Autodesk Inventor part; units mm, degrees
ref_plane "YZ Plane" through (0, 0, 0) normal (1, 0, 0) x (0, 1, 0)
ref_plane "XZ Plane" through (0, 0, 0) normal (0, 1, 0) x (-1, 0, 0)
ref_plane "XY Plane" through (0, 0, 0) normal (0, 0, 1) x (1, 0, 0)
sketch "Sketch1" plane through (0, 0, 0) normal (0, 1, 0) x (-1, 0, 0)
  line L0 (13.8415, 5.1768) -> (-89.2585, 5.1768)
  line L1 (-89.2585, 5.1768) -> (-89.2585, -12.8232)
  line L2 (-89.2585, -12.8232) -> (-79.2585, -12.8232)
  line L3 (-79.2585, -12.8232) -> (-79.2585, -4.5732)
  line L4 (-79.2585, -4.5732) -> (-0.8085, -4.5732)
  line L5 (-0.8085, -4.5732) -> (-0.8085, -11.3232)
  line L6 (-0.8085, -11.3232) -> (13.8415, -11.3232)
  line L7 (13.8415, -11.3232) -> (13.8415, 5.1768)
  circle A0 centre (2.4165, -8.8982) radius 1.325
  circle A1 centre (-83.9335, -9.1482) radius 1.325
  line L8 (13.8415, 5.1768) -> (-89.2585, 5.1768)
  line L9 (-89.2585, 5.1768) -> (-89.2585, 6.1768)
  line L10 (-89.2585, 6.1768) -> (13.8415, 6.1768)
  line L11 (13.8415, 6.1768) -> (13.8415, 5.1768)
  point P0 (0, 0)
  dimension "d0" = 2.65
  dimension "d1" = 2.65
  dimension "d2" = 103.1
  dimension "d3" = 14.65
  dimension "d4" = 10
  dimension "d5" = 18
  dimension "d6" = 16.5
  dimension "d7" = 14.075
  dimension "d8" = 11.425
  dimension "d9" = 9.75
  dimension "d10" = 14.325
  dimension "d11" = 5.325
  dimension "d14" = 1
extrude "Extrusion1" add sketch "Sketch1" along normal blind 1
extrude "Extrusion2" add sketch "Sketch1" against normal blind 7.6 contours L0 L9 L10 L11
sketch "Sketch3" plane through (89.2585, 0, 5.1768) normal (0, 0, -1) x (-1, 0, 0)
  line L0 (103.1, -7.6) -> (0, -7.6)
  line L1 (103.1, -7.6) -> (103.1, 1)
  line L2 (0, -7.6) -> (103.1, -7.6)
  line L3 (103.1, -7.6) -> (103.1, -6.6)
  line L4 (103.1, -6.6) -> (0, -6.6)
  line L5 (0, -6.6) -> (0, -7.6)
  point P0 (89.2585, 0)
  dimension "d17" = 1
extrude "Extrusion3" add sketch "Sketch3" along normal blind 19
sketch "Sketch4" plane through (0, 1, 0) normal (0, 1, 0) x (1, 0, 0)
  line L0 (79.2585, 4.5732) -> (0.8085, 4.5732)
  line L1 (18.2585, 4.5732) -> (33.2585, 4.5732)
  line L2 (33.2585, 4.5732) -> (33.2585, 0.3232)
  line L3 (33.2585, 0.3232) -> (18.2585, 0.3232)
  line L4 (18.2585, 0.3232) -> (18.2585, 4.5732)
  line L5 (0.8085, 4.5732) -> (0.8085, 11.3232)
  line L6 (79.2585, 12.8232) -> (79.2585, 4.5732)
  line L7 (-13.8415, -6.1768) -> (89.2585, -6.1768)
  point P0 (0, 0)
  point P1 (33.2585, 4.5732)
  dimension "d21" = 15
  dimension "d26" = 6.5
  dimension "d28" = 46
extrude "Extrusion4" cut sketch "Sketch4" against normal blind 2
properties part number "CO-1-03-jetsonMount"
Part model, mm, in its own coordinate system. A direction names the side the tool comes from. Round coordinates to 2 decimals unless told otherwise and drop trailing zeros. Loops run counter-clockwise (first coordinate to the right, second up) from the corner with the lowest first, then second, coordinate; pieces in that order, holes last. Notation, with made-up numbers: (-3.75, 47) - (5.25, 47) arc R26 cw to (5.25, 83) - close; hole circle Ø1 at (88.5, 19). An arc over 180 degrees is marked (long way). Answer as a JSON object with one key per item and string values.
Item 1: Pull direction Y, two halves, no side cores. Call faces 1 (the face through (38, 0, 0)), 2 (the face through (37, -6.6, -4)), 3 (the face through (38, 1, 1)), 4 (the face through (-13.842, -7, -2)): pulls with the +Y half, pulls with the -Y half, needs draft (parallel to the pull), parting line crosses it, or undercut.
Output:
{"face 1": "undercut", "face 2": "undercut", "face 3": "pulls with the +Y half", "face 4": "needs draft"}
Item 2: Band-saw the part on D-D on x = 53. List the corners of the cut face in (y, z), plus the area to 4 significant figures.
Output:
{"outline": "(-7.6, -13.82) - (-6.6, -13.82) - (-6.6, 5.18) - (0, 5.18) - (0, -4.57) - (1, -4.57) - (1, 6.18) - (-7.6, 6.18) - close", "area": "37.35 mm2"}
Item 3: Wall check: L1, parallel to X at y = 0.25, z = -9; L2, parallel to Y at x = -7, z = 4.25; L3, parallel to X at y = 0.25, z = -12. Give the ranges that are in metal, low to high.
Output:
{"L1": "-13.84 to -3.74, -1.1 to 0.81, 79.26 to 82.62, 85.25 to 89.26", "L2": "-7.6 to -6.6, 0 to 1", "L3": "79.26 to 89.26"}
Item 4: Tool access for faces 5 (the face through (83.322, 0.493, -7.973)), 6 (the face through (89.258, -7, -2)), 7 (the face through (37, -3, 5.177)): list every direction of +Z, -Z, +X, -X, +Y, -Y with a clear straight run to the whole face (end or side of a thin tool).
Output:
{"face 5": "+Y", "face 6": "+Z, -Z, +X, +Y, -Y", "face 7": "-Z, +X, -X"}
Item 5: Band-saw the part on A-A on z = -3.5. List the corners of the cut face in (x, y).
Output:
{"outline": "(-13.84, -7.6) - (89.26, -7.6) - (89.26, -6.6) - (-13.84, -6.6) - close; (-13.84, 0) - (18.26, 0) - (18.26, 1) - (-13.84, 1) - close; (33.26, 0) - (89.26, 0) - (89.26, 1) - (33.26, 1) - close"}
Item 6: Band-saw the part on B-B on z = 1. List the corners of the cut face in (x, y), plus the area to 3 significant figures.
Output:
{"outline": "(-13.84, -7.6) - (89.26, -7.6) - (89.26, -6.6) - (-13.84, -6.6) - close; (-13.84, 0) - (89.26, 0) - (89.26, 1) - (-13.84, 1) - close", "area": "206 mm2"}
Item 7: Band-saw the part on C-C on x = 28.5. List the corners of the cut face in (y, z).
Output:
{"outline": "(-7.6, -13.82) - (-6.6, -13.82) - (-6.6, 5.18) - (0, 5.18) - (0, -0.32) - (1, -0.32) - (1, 6.18) - (-7.6, 6.18) - close"}
Item 8: Pin check, flat tips, straight feed: pin 1 (4 mm diameter, centred on x = 56, y = -0.5, fed in from -Z); pin 2 (0.5 mm diameter, centred on x = 25, y = 0.5, fed in from -Z); pin 3 (2 mm diameter, centred on y = -3, z = 2.5, fed in from +X); pin 4 (2.5 mm diameter, centred on x = 83.93, z = -9.15, fed in from +Y). Stop position of each tip, or through.
Output:
{"pin 1": "z = -4.57", "pin 2": "z = -0.32", "pin 3": "through", "pin 4": "y = -6.6"}
